from build123d import *

# Parameters (mm, degrees)
SCHIZZO1_R                    = 7
ESTRUSIONE1_DEPTH             = 20
SCHIZZO2_R                    = 10
ESTRUSIONE2_DEPTH             = 226
SCHIZZO6_R                    = 13
ESTRUSIONE_ESTRUSIONE1_DEPTH  = 75
SCHIZZO7_R                    = 10
ESTRUSIONE_ESTRUSIONE2_DEPTH  = 93
FORO_FILETTATO_M10_1_D        = 8.5
FORO_FILETTATO_M10_1_DEPTH    = 27.5
FORO_FILETTATO_M10_1_TIP      = 2.553657631
TAGLIO_ESTRUSIONE1_DEPTH      = 10
TAGLIO_ESTRUSIONE1_DEPTH_BACK = 10
SCHIZZO10_R                   = 3.25


with BuildPart() as part:
    # Schizzo1 → Estrusione1 (new body)
    with BuildSketch(Plane.XY):
        Circle(SCHIZZO1_R)
    extrude(amount=ESTRUSIONE1_DEPTH)

    # Schizzo2 → Estrusione2 (add)
    with BuildSketch(Plane.XY.offset(20)):
        Circle(SCHIZZO2_R)
    extrude(amount=ESTRUSIONE2_DEPTH)

    # Schizzo6 → Estrusione-Estrusione1 (add)
    with BuildSketch(Plane.XY.offset(246)):
        Circle(SCHIZZO6_R)
    extrude(amount=ESTRUSIONE_ESTRUSIONE1_DEPTH)

    # Schizzo7 → Estrusione-Estrusione2 (add)
    with BuildSketch(Plane.XY.offset(321)):
        Circle(SCHIZZO7_R)
    extrude(amount=ESTRUSIONE_ESTRUSIONE2_DEPTH)

    # Foro filettato M10-1
    with Locations(Plane.XY.offset(414)):
        with Locations((0, 0)):
            Hole(FORO_FILETTATO_M10_1_D / 2, depth=FORO_FILETTATO_M10_1_DEPTH)
            with Locations((0, 0, -(FORO_FILETTATO_M10_1_DEPTH + FORO_FILETTATO_M10_1_TIP / 2))):  # 118° drill point
                Cone(0, FORO_FILETTATO_M10_1_D / 2, FORO_FILETTATO_M10_1_TIP, mode=Mode.SUBTRACT)

    # Schizzo10 → Taglio-Estrusione1 (cut, two sides: drawn at the far end of the back side and taken through both)
    with BuildSketch(Plane(origin=(0, 0, 0), x_dir=(1, 0, 0), z_dir=(0, 1, 0)).offset(-TAGLIO_ESTRUSIONE1_DEPTH_BACK)):
        with Locations(Location((0, -13.5, 0), (0, 0, 90))):
            Circle(SCHIZZO10_R)
    extrude(amount=TAGLIO_ESTRUSIONE1_DEPTH + TAGLIO_ESTRUSIONE1_DEPTH_BACK, mode=Mode.SUBTRACT)


solid = part.part
The model under review builds one solid part; all positions refer to its coordinate system, in mm. A direction names the side the tool comes from. Coordinates: 2 decimals unless noted, no trailing zeros. Put each result on its own line as item: value. Start each with the question number.
Q1. For faces 4 (the flat face through (7, -8, 246)), 5 (the flat face through (0, 0, 0)), 6 (the cylindrical face through (-2.17, -9.76, 366.85)), list the 3-axis set-ups (+Z, -Z, +X, -X, +Y, -Y) from which the entire face can be reached by the end or side of a thin tool; tool diameter is ignored.
Q2. Wall thickness on line 1 (Y direction, x = 0, z = 393); line 2 (Z direction, x = 4.25, y = 11.25); line 3 (X direction, y = 2, z = 13.5): over which ranges is each line inside the solid? List them lowest first.
Q3. Clearance check with flat-ended pins moving along their axes: pin 1 (5 mm diameter, centred on y = -3.5, z = 300.5, fed in from +X); pin 2 (7 mm diameter, centred on x = 0, y = 0, fed in from +Z); pin 3 (2 mm diameter, centred on x = 7, z = 176, fed in from +Y); pin 4 (6 mm diameter, centred on x = 0, z = 13.5, fed in from -Y). State where each tip first meets the part, or that it passes through.
Q4. The part is to be moulded in two halves that separate along X. For faces 1 (the flat face through (7, -8, 321)), 2 (the cylindrical face through (-2.17, -9.76, 131.42)), 3 (the cylindrical face through (-2.285, 3.584, 400.058)), say which applies: +X half, -X half, draft (parallel to the pull), parting line (faces both ways), or undercut.
Answers:
1. face 4: -Z
1. face 5: -Z, +X, -X, +Y, -Y
1. face 6: +Z
2. line 1: y = -10 to -4.25, 4.25 to 10
2. line 2: z = 246 to 321
2. line 3: x = -6.71 to -3.25, 3.25 to 6.71
3. pin 1: stops at x = 12.96
3. pin 2: stops at z = 386.05
3. pin 3: stops at y = 8
3. pin 4: passes through
4. face 1: draft
4. face 2: parting line
4. face 3: undercut
